```python
from build123d import *

# Parameters (mm, degrees)
CROQUIS2_R              = 1.45
SALIENTE_EXTRUIR1_DEPTH = 2.5
CROQUIS3_R              = 2.4
CROQUIS3_R_2            = 1.45
SALIENTE_EXTRUIR2_DEPTH = 3.5
CROQUIS4_R              = 1.69
CORTAR_EXTRUIR1_DEPTH   = 24.959444902


with BuildPart() as part:
    # Croquis2 → Saliente-Extruir1 (new body)
    with BuildSketch(Plane(origin=(0, 0, 0), x_dir=(1, 0, 0), z_dir=(0, 1, 0))):
        with BuildLine():
            Line((0, 3.45), (20, 3.45))
            ThreePointArc((20, 3.45), (23.45, 0), (20, -3.45))
            Line((20, -3.45), (0, -3.45))
            ThreePointArc((0, -3.45), (-3.45, 0), (0, 3.45))
        make_face()
        with Locations(Location((0, 0, 0), (0, 0, 270))):
            Circle(CROQUIS2_R, mode=Mode.SUBTRACT)
        with Locations(Location((10, 0, 0), (0, 0, 270))):
            Circle(CROQUIS2_R, mode=Mode.SUBTRACT)
    extrude(amount=SALIENTE_EXTRUIR1_DEPTH)

    # Croquis3 → Saliente-Extruir2 (add)
    # profile 1 of 2: a face of its own
    with BuildSketch(Plane(origin=(0, 2.5, 0), x_dir=(1, 0, 0), z_dir=(0, 1, 0))):
        with Locations(Location((0, 0, 0), (0, 0, 270))):
            Circle(CROQUIS3_R)
        with Locations(Location((0, 0, 0), (0, 0, 270))):
            Circle(CROQUIS3_R_2, mode=Mode.SUBTRACT)
    # profile 2 of 2: a face of its own
    with BuildSketch(Plane(origin=(0, 2.5, 0), x_dir=(1, 0, 0), z_dir=(0, 1, 0))):
        with Locations(Location((10, 0, 0), (0, 0, 270))):
            Circle(CROQUIS3_R)
        with Locations(Location((10, 0, 0), (0, 0, 270))):
            Circle(CROQUIS3_R_2, mode=Mode.SUBTRACT)
    extrude(amount=SALIENTE_EXTRUIR2_DEPTH)

    # Croquis4 → Cortar-Extruir1 (cut, through all)
    with BuildSketch(Plane(origin=(0, 2.5, 0), x_dir=(1, 0, 0), z_dir=(0, 1, 0))):
        with Locations(Location((20, 0, 0), (0, 0, 270))):
            Circle(CROQUIS4_R)
    extrude(amount=-CORTAR_EXTRUIR1_DEPTH, mode=Mode.SUBTRACT)


solid = part.part
```
Read the model definition and answer for the solid it produces. Units are mm, in the model's axes. A direction names the side the tool comes from. Coordinates: 2 decimals unless noted, no trailing zeros. Write each loop counter-clockwise with the first axis right and the second up, starting at its lowest first coordinate (ties: lowest second). Pieces come first, ordered by that corner, then holes. Notation, with made-up numbers: (19, -24) -> (48, -24) arc R18 cw to (48, 7) -> close; hole circle Ø8 at (25.25, 45.25). An arc over 180 degrees is marked (long way). Return JSON: item names as keys, results as strings.
1. A cutting plane is placed at C-C (y = 3.1). Determine the outline of the cut face in (x, z).
Found:
{"outline": "circle Ø4.8 at (0, 0); circle Ø4.8 at (10, 0); hole circle Ø2.9 at (0, 0); hole circle Ø2.9 at (10, 0)"}
2. Find the intervals of material crossed by line 1 along X through (y, z) = (1.25, 0); line 2 along X through (y, z) = (3.5, 0); line 3 along Y through (x, z) = (1.5, 2.75), in increasing order. Write a range as from..to.
Found:
{"line 1": "-3.45..-1.45, 1.45..8.55, 11.45..18.31, 21.69..23.45", "line 2": "-2.4..-1.45, 1.45..2.4, 7.6..8.55, 11.45..12.4", "line 3": "0..2.5"}
3. A cutting plane is placed at D-D (x = 14.5). Determine the outline of the cut face in (y, z), and give its area (4 significant figures).
Found:
{"outline": "(0, -3.45) -> (2.5, -3.45) -> (2.5, 3.45) -> (0, 3.45) -> close", "area": "17.25 mm2"}
4. A cutting plane is placed at B-B (x = 10). Determine the outline of the cut face in (y, z).
Found:
{"outline": "(0, -3.45) -> (2.5, -3.45) -> (2.5, -2.4) -> (6, -2.4) -> (6, -1.45) -> (0, -1.45) -> close; (0, 1.45) -> (6, 1.45) -> (6, 2.4) -> (2.5, 2.4) -> (2.5, 3.45) -> (0, 3.45) -> close"}
5. Determine the mould class of faces 1 (the face through (23.45, 1.23, -0.08)), 2 (the face through (8, 6, 0)), 3 (the face through (21.676, 1.268, -0.22)) for opening direction X: pulls with the +X half, pulls with the -X half, needs draft (parallel to the pull), parting line crosses it, or undercut.
Found:
{"face 1": "pulls with the +X half", "face 2": "needs draft", "face 3": "undercut"}
6. A tool of negligible diameter and unlimited length cuts with its end or side. For faces 4 (the face through (12.38, 4.23, -0.31)), 5 (the face through (10, 0, -2)), from which of +Z, -Z, +X, -X, +Y, -Y can it reach the whole face along a straight path? Write none if from no direction.
Found:
{"face 4": "+Y", "face 5": "+Z, -Z, +X, -X, -Y"}
7. Each of these flat-tipped pins is pushed along its axis until it touches: P1, Ø1, axis at y = 5, z = 1.5, coming from the -X side; P2, Ø1.5, axis at x = 6, y = 5, coming from the +Z side; P3, Ø2, axis at y = 4.5, z = -2, coming from the +X side; P4, Ø2, axis at x = 16, z = 1, coming from the +Y side. Where does it stop, or does it pass through?
Found:
{"P1": "x = -2.18", "P2": "through", "P3": "x = 12.18", "P4": "y = 2.5"}
8. A cutting plane is placed at A-A (z = 0). Determine the outline of the cut face in (x, y), and give its area (3 significant figures).
Found:
{"outline": "(-3.45, 0) -> (-1.45, 0) -> (-1.45, 6) -> (-2.4, 6) -> (-2.4, 2.5) -> (-3.45, 2.5) -> close; (1.45, 0) -> (8.55, 0) -> (8.55, 6) -> (7.6, 6) -> (7.6, 2.5) -> (2.4, 2.5) -> (2.4, 6) -> (1.45, 6) -> close; (11.45, 0) -> (18.31, 0) -> (18.31, 2.5) -> (12.4, 2.5) -> (12.4, 6) -> (11.45, 6) -> close; (21.69, 0) -> (23.45, 0) -> (23.45, 2.5) -> (21.69, 2.5) -> close", "area": "57.6 mm2"}
